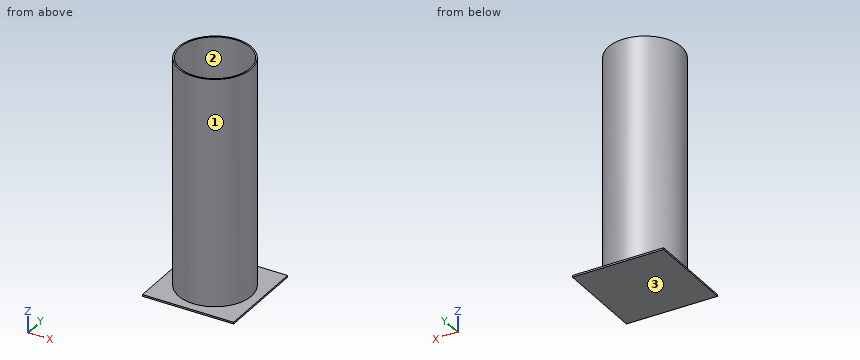
```python
from build123d import *

# Parameters (mm, degrees)
F0_R     = 101.6
F0_R_2   = 97.536
F1_DEPTH = 635
F2_W     = 254
F2_H     = 254
F3_DEPTH = 4.7625


with BuildPart() as f1:
    # F0 (on Top) → F1 (new body)
    with BuildSketch(Plane.XY):
        Circle(F0_R)
        Circle(F0_R_2, mode=Mode.SUBTRACT)
    extrude(amount=F1_DEPTH)

    # F2 (on Top) → F3 (join)
    with BuildSketch(Plane.XY):
        Rectangle(F2_W, F2_H)
    extrude(amount=-F3_DEPTH)


solid = f1.part
```
Part model, mm, in its own coordinate system. Face numbers are marked on the shaded views. Round coordinates to 2 decimals unless told otherwise and drop trailing zeros. Write each loop counter-clockwise with the first axis right and the second up, starting at its lowest first coordinate (ties: lowest second). Pieces come first, ordered by that corner, then holes. Notation, with made-up numbers: M -25.75,73 L 27.25,73 A29 cw 27.25,108 Z; hole C 88,59 d8. An arc over 180 degrees is marked long. One line per question, with ' | ' between items.
(1) Probe line 1 along X through (y, z) = (-1.5, 473); line 2 along Y through (x, z) = (0, 328); line 3 along Z through (x, y) = (2.5, 24.5). List the from-to ranges inside material, lowest first.
Answer key:
line 1: x = -101.59 to -97.52, 97.52 to 101.59 | line 2: y = -101.6 to -97.54, 97.54 to 101.6 | line 3: z = -4.76 to 0
(2) Saw through at C-C on z = 348.5. Write the cut outline in (x, y).
Answer key:
outline: C 0,0 d203.2; hole C 0,0 d195.07
(3) Pin check, flat tips, straight feed: pin 1 (3 mm diameter, centred on x = -12, z = 160.5, fed in from +Y); pin 2 (10 mm diameter, centred on y = -25, z = 165, fed in from +X); pin 3 (1.5 mm diameter, centred on y = 56, z = 117, fed in from +X). Stop position of each tip, or through.
Answer key:
pin 1: stops at y = 101.06 | pin 2: stops at x = 99.61 | pin 3: stops at x = 85.26
(4) Two-plate mould, pull along Y, no slides. Class the marked faces 1, 2 and 3: released by +Y, released by -Y, zero draft, split by the parting line, or undercut.
Answer key:
face 1: split by the parting line | face 2: undercut | face 3: zero draft
(5) Saw through at A-A on x = 0. Write the cut outline in (y, z).
Answer key:
outline: M -127,-4.76 L 127,-4.76 L 127,0 L 101.6,0 L 101.6,635 L 97.54,635 L 97.54,0 L -97.54,0 L -97.54,635 L -101.6,635 L -101.6,0 L -127,0 Z
